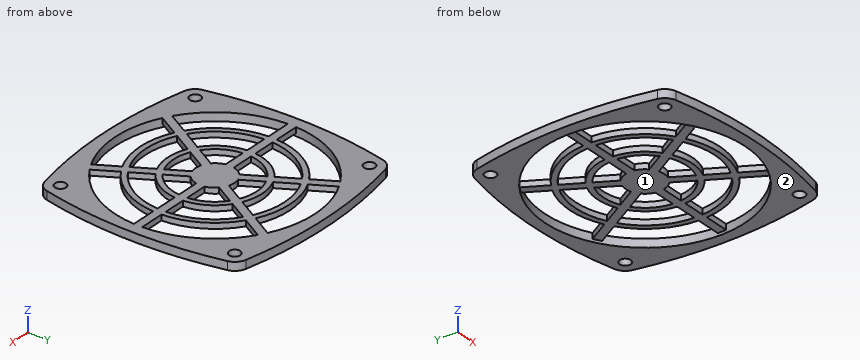
Autodesk Inventor part; units mm, degrees
ref_plane "YZ Plane" through (0, 0, 0) normal (1, 0, 0) x (0, 1, 0)
ref_plane "XZ Plane" through (0, 0, 0) normal (0, 1, 0) x (-1, 0, 0)
ref_plane "XY Plane" through (0, 0, 0) normal (0, 0, 1) x (1, 0, 0)
sketch "Эскиз1" plane through (0, 0, 0) normal (0, 0, 1) x (1, 0, 0)
  line L0 (-31.5, 31.5) -> (31.5, 31.5) construction
  line L1 (31.5, 31.5) -> (31.5, -31.5) construction
  line L2 (31.5, -31.5) -> (-31.5, -31.5) construction
  line L3 (-31.5, -31.5) -> (-31.5, 31.5) construction
  arc A0 (-32.5976, 36.378) -> (-36.378, 32.5976) centre (-31.5, 31.5) ccw
  line L4 (-40, 40) -> (40, 40) construction
  line L5 (40, 40) -> (40, -40) construction
  line L6 (40, -40) -> (-40, -40) construction
  line L7 (-40, -40) -> (-40, 40) construction
  arc A1 (-36.378, 32.5976) -> (-36.378, -32.5976) centre (108.5, 0) ccw
  line L8 (-40, 0) -> (40, 0)
  line L9 (0, 40) -> (0, -40)
  arc A2 (32.5976, 36.378) -> (-32.5976, 36.378) centre (0, -108.5) ccw
  arc A3 (36.378, 32.5976) -> (32.5976, 36.378) centre (31.5, 31.5) ccw
  arc A4 (-36.378, -32.5976) -> (-32.5976, -36.378) centre (-31.5, -31.5) ccw
  arc A5 (-32.5976, -36.378) -> (32.5976, -36.378) centre (0, 108.5) ccw
  arc A6 (36.378, -32.5976) -> (36.378, 32.5976) centre (-108.5, 0) ccw
  circle A7 centre (0, 0) radius 36
  circle A8 centre (-31.5, 31.5) radius 2
  circle A9 centre (31.5, 31.5) radius 2
  circle A10 centre (31.5, -31.5) radius 2
  circle A11 centre (-31.5, -31.5) radius 2
  arc A12 (32.5976, -36.378) -> (36.378, -32.5976) centre (31.5, -31.5) ccw
  point P0 (0, 31.5)
  point P1 (31.5, 0)
  dimension "d0" = 63
  dimension "d1" = 5
  dimension "d2" = 80
  dimension "d3" = 72
  dimension "d4" = 4
extrude "Выдавливание1" add sketch "Эскиз1" along normal blind 3 contours A2 L9 A7 L8 A1 A0 | A2 A3 A6 L8 A7 L9 | L8 A7 L9 A5 A4 A1 | L8 A6 A12 A5 L9 A7
sketch "Эскиз2" plane through (0, 0, 3) normal (0, 0, 1) x (1, 0, 0)
  circle A0 centre (0, 0) radius 5
  circle A1 centre (0, 0) radius 7
  circle A2 centre (0, 0) radius 15
  circle A3 centre (0, 0) radius 17
  circle A4 centre (0, 0) radius 27
  circle A5 centre (0, 0) radius 25
  circle A6 centre (0, 0) radius 36
  dimension "d7" = 2
  dimension "d8" = 2
  dimension "d9" = 2
  dimension "d10" = 10
  dimension "d11" = 30
  dimension "d12" = 50
extrude "Выдавливание2" add sketch "Эскиз2" against normal blind 2 contours A1 | A3 | A4
sketch "Эскиз3" plane through (0, 0, 3) normal (0, 0, 1) x (1, 0, 0)
  line L0 (-39.9924, 1.5) -> (-6.8374, 1.5)
  line L1 (-6.8374, 1.5) -> (-6.8374, -1.5)
  line L2 (-6.8374, -1.5) -> (-39.9924, -1.5)
  line L3 (-39.9924, -1.5) -> (-39.9924, 1.5)
  circle A0 centre (0, 0) radius 7
  arc A1 (-36.378, 32.5976) -> (-36.378, -32.5976) centre (108.5, 0) ccw
  dimension "d15" = 3
extrude "Выдавливание3" add sketch "Эскиз3" against normal blind 2 contours L0 A0 L2 L3 | A0 L1 | L1 A0
pattern_circular "Круговой массив1" count 6 over 360 about axis through (0, 0, -10) along (0, 0, 1) of "Выдавливание3"
properties part number "Speaker_Secure"
Input: part model. Units: mm. Frame: model coordinates. Face numbers are marked on the shaded views. Give positions to 0.01 mm unless a question says otherwise; leave off trailing zeros. Write each loop counter-clockwise with the first axis right and the second up, starting at its lowest first coordinate (ties: lowest second). Pieces come first, ordered by that corner, then holes. Notation, with made-up numbers: M 46.5,22 L 54.5,22 A20 cw 54.5,61 Z; hole C 64.25,20.25 d2. An arc over 180 degrees is marked long. Use one line per item in the form item = value.
1. Cut plane B-B on y = -2.5. Return loops of the section in (x, z).
Outcome:
outline = M -39.98,0 L -35.91,0 L -35.91,3 L -39.98,3 Z; M -26.88,1 L -24.87,1 L -24.87,3 L -26.88,3 Z; M -16.82,1 L -14.79,1 L -14.79,3 L -16.82,3 Z; M -6.54,1 L 6.54,1 L 6.54,3 L -6.54,3 Z; M 14.79,1 L 16.82,1 L 16.82,3 L 14.79,3 Z; M 24.87,1 L 26.88,1 L 26.88,3 L 24.87,3 Z; M 35.91,0 L 39.98,0 L 39.98,3 L 35.91,3 Z
2. Cut plane D-D on z = 2. State how many separate pieces and enclosed holes the cut face has, and give its area (3 significant figures).
Outcome:
separate_pieces = 1
enclosed_holes = 22
area = 2,920 mm²
3. Cut plane C-C on x = -31.5. Return loops of the section in (y, z), and give its area (3 significant figures).
Outcome:
outline = M -36.62,0 L -33.5,0 L -33.5,3 L -36.62,3 Z; M -29.5,0 L -17.43,0 L -17.43,3 L -29.5,3 Z; M -1.5,1 L 1.5,1 L 1.5,3 L -1.5,3 Z; M 17.43,0 L 29.5,0 L 29.5,3 L 17.43,3 Z; M 33.5,0 L 36.62,0 L 36.62,3 L 33.5,3 Z
area = 97.2 mm²
4. Ray query, L1, parallel to Y at x = 31.5, z = 0.8; L2, parallel to Y at x = -31.5, z = 1.85; L3, parallel to X at y = -27.5, z = 2.8. Return the intervals inside material, ascending.
Outcome:
L1 = -36.62 to -33.5, -29.5 to -17.43, 17.43 to 29.5, 33.5 to 36.62
L2 = -36.62 to -33.5, -29.5 to -17.43, -1.5 to 1.5, 17.43 to 29.5, 33.5 to 36.62
L3 = -37.43 to -23.23, -17.61 to -14.15, 14.15 to 17.61, 23.23 to 37.43
5. Cut plane A-A on x = 0. Return loops of the section in (y, z), and give its area (3 significant figures).
Outcome:
outline = M -40,0 L -36,0 L -36,3 L -40,3 Z; M -27,1 L -25,1 L -25,3 L -27,3 Z; M -17,1 L -15,1 L -15,3 L -17,3 Z; M -7,1 L 7,1 L 7,3 L -7,3 Z; M 15,1 L 17,1 L 17,3 L 15,3 Z; M 25,1 L 27,1 L 27,3 L 25,3 Z; M 36,0 L 40,0 L 40,3 L 36,3 Z
area = 68.0 mm²
6. First-contact query: P1, Ø1, axis at x = 31.5, z = 2, coming from the -Y side; P2, Ø0.6, axis at x = 10, z = 1.5, coming from the -Y side; P3, Ø1.5, axis at x = 0.5, z = 2.5, coming from the -Y side. Flat tips, straight axial feed; report the tip coordinate or a pass-through.
Outcome:
P1 = -36.73
P2 = -39.68
P3 = -40
7. Mould query, pull axis X, two halves, no side actions, for the marked faces 1 and 2. Classes: released by +X, released by -X, zero draft, split by the parting line, or undercut.
Outcome:
face_1 = undercut
face_2 = zero draft
